The listing builds one solid part. Answer for the finished solid, in the listing's coordinates (mm). Coordinates: 2 decimals unless noted, no trailing zeros. Loops run counter-clockwise (first coordinate to the right, second up) from the corner with the lowest first, then second, coordinate; pieces in that order, holes last. Notation, with made-up numbers: M 10.25,-37 L 52.25,-37 A25 cw 52.25,-25 Z; hole C -8.75,-15 d1. An arc over 180 degrees is marked long. Answer as CSV lines item,"result". Start each with the question number.
```python
from build123d import *

# Parameters (mm, degrees)
F0_R     = 32.8
F0_R_2   = 26.15
F2_DEPTH = 1.5
F1_W     = 2.5
F1_H     = 5
F3_DEPTH = 3.25
F4_COUNT = 24


with BuildPart() as f2:
    # F0 (on Top) → F2 (new body)
    with BuildSketch(Plane.XY):
        Circle(F0_R)
        Circle(F0_R_2, mode=Mode.SUBTRACT)
    extrude(amount=F2_DEPTH)

    # F1 (on Top) → F3 (join)
    with BuildSketch(Plane.XY):
        with Locations((-1.25, 29.475)):
            Rectangle(F1_W, F1_H)
        with Locations((1.25, 29.475)):
            Rectangle(F1_W, F1_H)
    extrude(amount=F3_DEPTH)

    # F4: F2 ×24 about axis
    f4_axis = Axis((0, 0, 0), (0, 0, 1))


with BuildPart() as f2_1:
    add(f2.part)
    for i in range(1, F4_COUNT):
        add(f2.part.rotate(f4_axis, i * 360 / F4_COUNT))


solid = f2_1.part
```
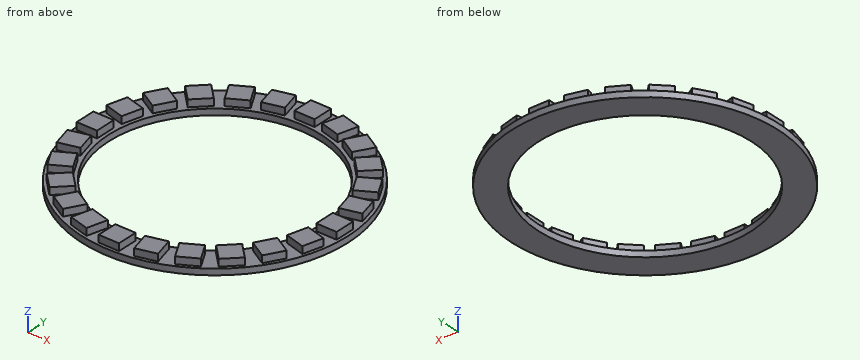
Item 1: Section A-A on x = 0 is taken. Determine the outline of the cut face in (y, z) (3 decimals).
Item 2: Consider line 1 (Y direction, x = 0, z = 0.5); line 2 (X direction, y = 28, z = 2.1); line 3 (Y direction, x = -30, z = 1.7). Determine where each line is inside the solid, lowest interval first.
Item 3: Each of these flat-tipped pins is pushed along its axis until it touches: P1, Ø0.5, axis at y = 0.5, z = 2.5, coming from the +X side (3 decimals); P2, Ø1.4, axis at y = 28.5, z = 2.5, coming from the -X side; P3, Ø1.9, axis at x = 0.5, z = 2.5, coming from the -Y side (3 decimals). Where does it stop, or does it pass through?
Item 4: Section C-C on z = 1 is taken. Determine the outline of the cut face in (x, y), then the cut area to 3 significant figures.
Results are:
1,outline,"M -32.8,0 L -26.15,0 L -26.15,1.5 L -26.975,1.5 L -26.975,3.25 L -31.975,3.25 L -31.975,1.5 L -32.8,1.5 Z; M 26.15,0 L 32.8,0 L 32.8,1.5 L 31.975,1.5 L 31.975,3.25 L 26.975,3.25 L 26.975,1.5 L 26.15,1.5 Z"
2,line 1,"-32.8 to -26.15, 26.15 to 32.8"
2,line 2,"-15.45 to -13.28, -10.09 to -4.91, -2.5 to 2.5, 4.91 to 10.09, 13.28 to 15.45"
2,line 3,"-10.63 to -5.45, -2.5 to 2.5, 5.45 to 10.63"
3,P1,"x = 31.975"
3,P2,"x = -15.8"
3,P3,"y = -31.975"
4,outline,"C 0,0 d65.6; hole C 0,0 d52.3"
4,area,"1,230 mm²"
